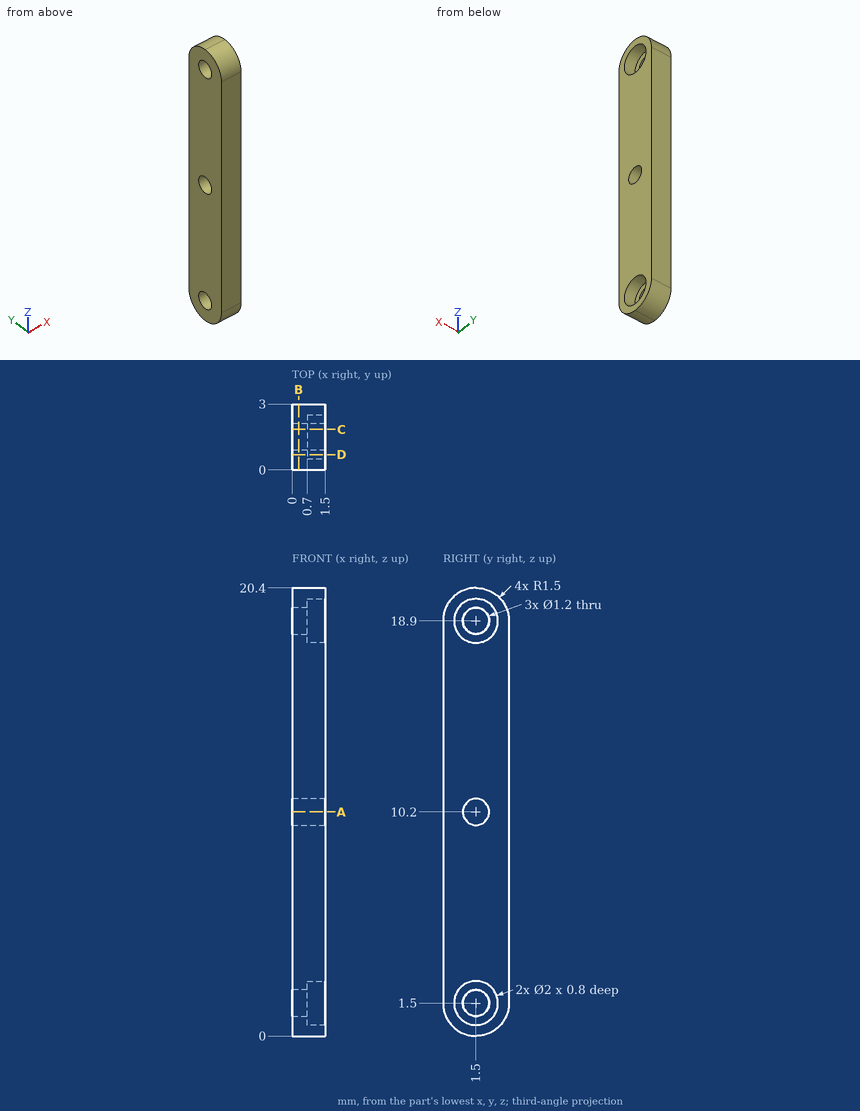
Can you work these out from the drawing? Everything is in mm from the part's minimum corner. Coordinates: 2 decimals unless noted, no trailing zeros. Order: outer loops, then holes, each group sorted by start corner. A loop starts at its lowest first (then second) coordinate and runs counter-clockwise, first axis right, second up. Notation, with made-up numbers: (66, 28) -> (71, 28) arc R22 ccw to (71, 67) -> close; hole circle Ø4 at (59, -35.5). An arc over 180 degrees is marked (long way). Use one line per item in the form item = value.
Q1. Will these pins go through, and if not, where does the flat tip stop? P1, Ø1.6, axis at y = 1.5, z = 18.9, coming from the +X side; P2, Ø0.7, axis at y = 1.5, z = 18.9, coming from the -X side.
From the geometry:
P1 = 0.7
P2 = through
Q2. Imagine slicing it at D-D, the plane y = 0.7. List the corners of the cut face in (x, z) for me, then the cut area to 3 significant figures.
From the geometry:
outline = (0, 0.23) -> (1.5, 0.23) -> (1.5, 0.9) -> (0.7, 0.9) -> (0.7, 2.1) -> (1.5, 2.1) -> (1.5, 18.3) -> (0.7, 18.3) -> (0.7, 19.5) -> (1.5, 19.5) -> (1.5, 20.17) -> (0, 20.17) -> close
area = 28.0 mm²
Q3. I need wall thicknesses on L1, parallel to Y at x = 1.15, z = 10.2; L2, parallel to Z at x = 0.75, y = 2.3; L3, parallel to Y at x = 1.3, z = 1.5. Which ranges of each line are inside material? Lowest first, please.
From the geometry:
L1 = 0 to 0.9, 2.1 to 3
L2 = 0.23 to 0.9, 2.1 to 18.3, 19.5 to 20.17
L3 = 0 to 0.5, 2.5 to 3
Q4. Imagine slicing it at C-C, the plane y = 1.85. List the corners of the cut face in (x, z) for me.
From the geometry:
outline = (0, 0.04) -> (1.5, 0.04) -> (1.5, 0.56) -> (0.7, 0.56) -> (0.7, 1.01) -> (0, 1.01) -> close; (0, 1.99) -> (0.7, 1.99) -> (0.7, 2.44) -> (1.5, 2.44) -> (1.5, 9.71) -> (0, 9.71) -> close; (0, 10.69) -> (1.5, 10.69) -> (1.5, 17.96) -> (0.7, 17.96) -> (0.7, 18.41) -> (0, 18.41) -> close; (0, 19.39) -> (0.7, 19.39) -> (0.7, 19.84) -> (1.5, 19.84) -> (1.5, 20.36) -> (0, 20.36) -> close
Q5. Imagine slicing it at B-B, the plane x = 0.3. Give the number of separate pieces and of enclosed holes in the cut face, then the cut area to 3 significant figures.
From the geometry:
separate_pieces = 1
enclosed_holes = 3
area = 55.9 mm²
Q6. Imagine slicing it at A-A, the plane z = 10.2. List the corners of the cut face in (x, y) for me.
From the geometry:
outline = (0, 0) -> (1.5, 0) -> (1.5, 0.9) -> (0, 0.9) -> close; (0, 2.1) -> (1.5, 2.1) -> (1.5, 3) -> (0, 3) -> close
